For this review, take the finished solid that the model builds, in its own axes (mm). A direction names the side the tool comes from. Give positions to 0.01 mm unless a question says otherwise; leave off trailing zeros. Loops run counter-clockwise (first coordinate to the right, second up) from the corner with the lowest first, then second, coordinate; pieces in that order, holes last. Notation, with made-up numbers: M -35,67.25 L 2,67.25 A35 ccw 2,102.25 Z; hole C 28.5,42.25 d9. An arc over 180 degrees is marked long. Use CSV: the item, a comma, the result in double quotes. Start each with the question number.
1. Take a section at A-A, the plane y = 29. Write out the cut boundary in (x, z).
2. Take a section at B-B, the plane x = 13. Write out the cut boundary in (y, z).
3. Insertion check: P1, Ø14, axis at x = 10.5, z = 7, coming from the -Y side; P2, Ø6, axis at x = 17, z = -2, coming from the +Y side; P3, Ø6, axis at x = -2.5, z = 14.5, coming from the +Y side. Each pin has a flat end and moves straight along its axis. Give the tip position at first contact, or say it passes through.
4. Tool access review of faces 1 (the face through (-2, 8, 0)), 2 (the face through (-6, 8, -5)), 3 (the face through (30, 7.9, -2.5)), 4 (the face through (13, 36, 15)), 5 (the face through (3, 8, -5)): name each direction out of +Z, -Z, +X, -X, +Y, -Y from which nothing blocks a thin tool from reaching the whole face with its end or side.
5. To check wall thickness, follow line 1 (Y direction, x = 13, z = 17.7); line 2 (Z direction, x = 8.5, y = 5.5); line 3 (Z direction, x = 3, y = 7.5). State the ranges of each line that lie inside material, in increasing order. Write a range as [from, to].
6. Take a section at C-C, the plane y = 7.5. Write out the cut boundary in (x, z), and give its area (3 significant figures).
7. Take a section at D-D, the plane x = 30. Write out the cut boundary in (y, z).
8. The part is to be moulded in two halves that separate along X. For faces 6 (the face through (8, 32, 0)), 7 (the face through (16, 7.9, -2.5)), 8 (the face through (3, 32, -5)), 9 (the face through (29.99, 2.85, 17.46)), say which applies: pulls with the +X half, pulls with the -X half, needs draft (parallel to the pull), parting line crosses it, or undercut.
from build123d import *

# Parameters (mm, degrees)
BOSS_EXTRUDE1_DEPTH      = 40
SKETCH2_W                = 40
SKETCH2_H                = 3
BOSS_EXTRUDE2_DEPTH      = 60
BOSS_EXTRUDE3_DEPTH      = 15
BOSS_EXTRUDE3_DEPTH_BACK = 10
SKETCH3_W                = 40
SKETCH3_H                = 8
SKETCH4_W                = 40
SKETCH4_H                = 5
BOSS_EXTRUDE4_DEPTH      = 40
SKETCH5_R                = 2.5
CUT_EXTRUDE1_DEPTH       = 40
FILLET1_R                = 10
FILLET2_R                = 2.5
FILLET3_START            = -7
FILLET3_DEPTH            = 40
FILLET4_R                = 2


with BuildPart() as part:
    # Sketch1 → Boss-Extrude1 (new body)
    with BuildSketch(Plane(origin=(0, 0, 0), x_dir=(1, 0, 0), z_dir=(0, 1, 0))):
        Polygon((-7, 10), (-7, 5), (-5, 5), (-3, 0), (-1, 0), (1, 5), (5, 5), (7, 0), (9, 0), (11, 5), (15, 5), (17, 0), (19, 0), (21, 5), (25, 5), (27, 0), (29, 0), (31, 5), (33, 5), (33, 10), (31.5, 10), align=None)
    extrude(amount=BOSS_EXTRUDE1_DEPTH)

    # Sketch2 → Boss-Extrude2 (add)
    with BuildSketch(Plane(origin=(0, 0, 0), x_dir=(1, 0, 0), z_dir=(0, 1, 0))):
        with Locations((13, 8.5)):
            Rectangle(SKETCH2_W, SKETCH2_H)
    extrude(amount=BOSS_EXTRUDE2_DEPTH)

    # Sketch3 → Boss-Extrude3 (add, two sides: drawn at the far end of the back side and taken through both)
    with BuildSketch(Plane.XY.offset(-BOSS_EXTRUDE3_DEPTH_BACK)):
        with Locations((13, 20)):
            Rectangle(SKETCH3_W, SKETCH3_H)
    extrude(amount=BOSS_EXTRUDE3_DEPTH + BOSS_EXTRUDE3_DEPTH_BACK)

    # Sketch4 → Boss-Extrude4 (add)
    with BuildSketch(Plane(origin=(0, 0, 0), x_dir=(1, 0, 0), z_dir=(0, 1, 0))):
        with Locations((13, -17.5)):
            Rectangle(SKETCH4_W, SKETCH4_H)
    extrude(amount=BOSS_EXTRUDE4_DEPTH)

    # Sketch5 → Cut-Extrude1 (cut)
    with BuildSketch(Plane.XY.offset(10)):
        with Locations(Location((13, 32.5, 0), (0, 0, 180))):
            Circle(SKETCH5_R)
        with Locations(Location((13, 7.5, 0), (0, 0, 180))):
            Circle(SKETCH5_R)
    extrude(amount=CUT_EXTRUDE1_DEPTH, mode=Mode.SUBTRACT)

    # Fillet1
    fillet1_edges = [part.edges().sort_by_distance(p)[0] for p in [
        (-7, 0, 17.5),
        (33, 0, 17.5),
        (33, 40, 17.5),
        (-7, 40, 17.5),
    ]]
    fillet(fillet1_edges, radius=FILLET1_R)

    # Fillet2
    fillet2_edges = [part.edges().sort_by_distance(p)[0] for p in [
        (13, 16, 15),
        (13, 24, 15),
    ]]
    fillet(fillet2_edges, radius=FILLET2_R)

    # Fillet3: read off the stored shape, not the designer's step
    # Fillet3 outline → Fillet3 (add)
    with BuildSketch(Plane.YZ.offset(FILLET3_START)):
        with BuildLine():
            Line((40, -7), (42, -7))
            ThreePointArc((42, -7), (40.585786438, -6.414213562), (40, -5))
            Line((40, -5), (40, -7))
        make_face()
    extrude(amount=FILLET3_DEPTH)

    # Fillet4
    fillet4_edges = [part.edges().sort_by_distance(p)[0] for p in [
        (-7, 60, -8.5),
        (33, 60, -8.5),
    ]]
    fillet(fillet4_edges, radius=FILLET4_R)


solid = part.part
Result set:
1,outline,"M -7,-10 L 33,-10 L 33,-5 L 31,-5 L 29,0 L 27,0 L 25,-5 L 21,-5 L 19,0 L 17,0 L 15,-5 L 11,-5 L 9,0 L 7,0 L 5,-5 L 1,-5 L -1,0 L -3,0 L -5,-5 L -7,-5 Z; M -7,15 L 33,15 L 33,20 L -7,20 Z"
2,outline,"M 0,-10 L 60,-10 L 60,-7 L 42,-7 A2 cw 40,-5 L 24,-5 L 24,12.5 A2.5 cw 26.5,15 L 30,15 L 30,20 L 10,20 L 10,15 L 13.5,15 A2.5 cw 16,12.5 L 16,-5 L 0,-5 Z; M 0,15 L 5,15 L 5,20 L 0,20 Z; M 35,15 L 40,15 L 40,20 L 35,20 Z"
3,P1,"y = 15.5"
3,P2,"y = 40"
3,P3,"y = 39.67"
4,face 1,"+X, -X, -Y"
4,face 2,"-X, -Y"
4,face 3,"+X, -Y"
4,face 4,"+X, -X, +Y"
4,face 5,"-Y"
5,line 1,"[0, 5], [10, 30], [35, 40]"
5,line 2,"[-10, 0], [15, 20]"
5,line 3,"[-10, -5], [15, 20]"
6,outline,"M -7,-10 L 33,-10 L 33,-5 L 31,-5 L 29,0 L 27,0 L 25,-5 L 21,-5 L 19,0 L 17,0 L 15,-5 L 11,-5 L 9,0 L 7,0 L 5,-5 L 1,-5 L -1,0 L -3,0 L -5,-5 L -7,-5 Z; M -6.68,15 L 10.5,15 L 10.5,20 L -6.68,20 Z; M 15.5,15 L 32.68,15 L 32.68,20 L 15.5,20 Z"
6,area,"452 mm2"
7,outline,"M 0,-10 L 60,-10 L 60,-7 L 42,-7 A2 cw 40,-5 L 40,-2.5 L 24,-2.5 L 24,12.5 A2.5 cw 26.5,15 L 37.14,15 L 37.14,20 L 2.86,20 L 2.86,15 L 13.5,15 A2.5 cw 16,12.5 L 16,-2.5 L 0,-2.5 Z"
8,face 6,"needs draft"
8,face 7,"undercut"
8,face 8,"undercut"
8,face 9,"pulls with the +X half"
